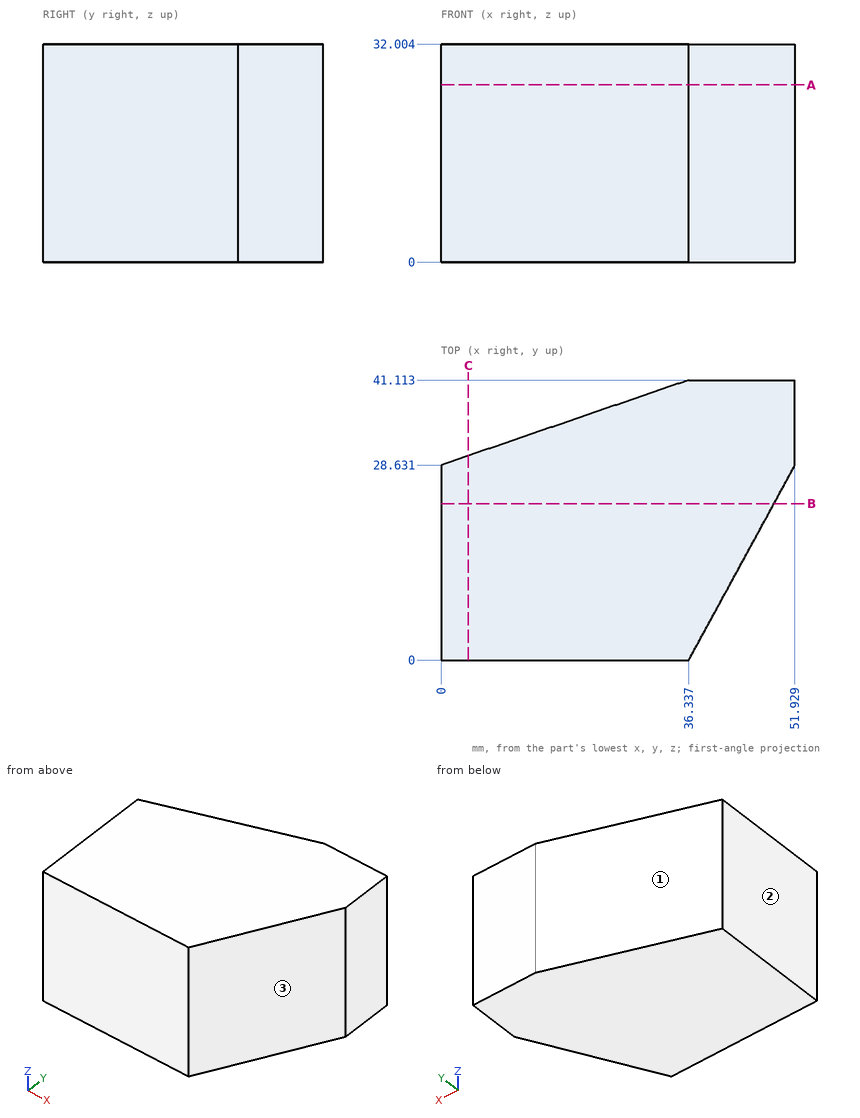
Drawing for the job (mm, zero at the part's lowest x, y, z). Coordinates: 2 decimals unless noted, no trailing zeros. Write each loop counter-clockwise with the first axis right and the second up, starting at its lowest first coordinate (ties: lowest second). Pieces come first, ordered by that corner, then holes. Notation, with made-up numbers: (68, -35.5) -> (90, -35.5) arc R25 cw to (90, -15.5) -> close; hole circle Ø4 at (22, -31). An arc over 180 degrees is marked (long way). One line per item, written item: value. Start each with the question number.
1) Slice it at A-A on z = 26. Write the cut outline in (x, y), then the cut area to 4 significant figures.
2) Slice it at B-B on y = 23. Write the cut outline in (x, z).
3) Pull direction Y, two halves, no side cores. Call the marked faces 1, 2 and 3: +Y half, -Y half, draft (parallel to the pull), parting line (faces both ways), or undercut.
4) Flat gauge pins, fed straight in: pin 1 Ø4 at (x, z) = (15.5, 15.5) entering from +Y; pin 2 Ø1 at (x, z) = (46.5, 23.5) entering from -Y (1 decimal). Where does each tip first touch, or does it go through?
5) Probe probe 1 along X at (y, z) = (13, 30) (1 decimal); probe 2 along X at (y, z) = (27.5, 19.5) (1 decimal); probe 3 along Y at (x, z) = (9, 6.5). List the from-to ranges inside material, lowest first.
6) Slice it at C-C on x = 4. Write the cut outline in (y, z) (1 decimal).
Answers follow:
1. outline: (0, 0) -> (36.34, 0) -> (51.93, 28.63) -> (51.93, 41.11) -> (36.34, 41.11) -> (0, 28.63) -> close
1. area: 1,685 mm2
2. outline: (0, 0) -> (48.86, 0) -> (48.86, 32) -> (0, 32) -> close
3. face 1: +Y half
3. face 2: draft
3. face 3: -Y half
4. pin 1: y = 34.64
4. pin 2: y = 17.7
5. probe 1: 0 to 43.4
5. probe 2: 0 to 51.3
5. probe 3: 0 to 31.72
6. outline: (0, 0) -> (30, 0) -> (30, 32) -> (0, 32) -> close
